Autodesk Inventor part; units mm, degrees
ref_plane "YZ Plane" through (0, 0, 0) normal (1, 0, 0) x (0, 1, 0)
ref_plane "XZ Plane" through (0, 0, 0) normal (0, 1, 0) x (-1, 0, 0)
ref_plane "XY Plane" through (0, 0, 0) normal (0, 0, 1) x (1, 0, 0)
sketch "Sketch1" plane through (0, 0, 0) normal (0, 1, 0) x (-1, 0, 0)
  line L0 (-90.805, 38.735) -> (90.805, 38.735)
  line L1 (90.805, 38.735) -> (90.805, -38.735)
  line L2 (90.805, -38.735) -> (-90.805, -38.735)
  line L3 (-90.805, -38.735) -> (-90.805, 38.735)
  line L4 (-90.805, 38.735) -> (90.805, -38.735) construction
  line L5 (90.805, 38.735) -> (-90.805, -38.735) construction
  line L6 (96.52, 43.18) -> (-96.52, 43.18)
  line L7 (-96.52, 43.18) -> (-96.52, -43.18)
  line L8 (-96.52, -43.18) -> (96.52, -43.18)
  line L9 (96.52, -43.18) -> (96.52, 43.18)
  line L10 (96.52, 43.18) -> (-96.52, -43.18) construction
  line L11 (-96.52, 43.18) -> (96.52, -43.18) construction
  point P0 (0, 0)
  dimension "d0" = 181.61
  dimension "d1" = 77.47
  dimension "d2" = 193.04
  dimension "d3" = 86.36
extrude "Extrusion1" add sketch "Sketch1" against normal blind 5.08 contours L0 L1 L2 L3 | L9 L8 L7 L6
extrude "Extrusion2" add sketch "Sketch1" along normal blind 83.566
sketch "Sketch2" plane through (-96.52, -5.08, 43.18) normal (0, 0, 1) x (1, 0, 0)
  line L0 (187.325, 88.646) -> (5.715, 88.646)
  line L1 (193.04, 88.646) -> (193.04, 0)
  line L2 (7.62, 82.423) -> (185.42, 82.423)
  line L3 (185.42, 82.423) -> (185.42, 6.223)
  line L4 (185.42, 6.223) -> (7.62, 6.223)
  line L5 (7.62, 6.223) -> (7.62, 82.423)
  line L6 (185.42, 50.673) -> (185.42, 37.973)
  line L7 (7.62, 37.973) -> (7.62, 50.673)
  line L8 (90.17, 82.423) -> (102.87, 82.423)
  line L9 (102.87, 6.223) -> (90.17, 6.223)
  line L10 (7.62, 50.673) -> (85.5215, 50.673)
  line L11 (107.5185, 50.673) -> (185.42, 50.673)
  line L12 (90.17, 6.223) -> (90.17, 33.3245)
  line L13 (90.17, 55.3215) -> (90.17, 82.423)
  line L14 (185.42, 37.973) -> (107.5185, 37.973)
  line L15 (85.5215, 37.973) -> (7.62, 37.973)
  line L16 (102.87, 82.423) -> (102.87, 55.3215)
  line L17 (102.87, 33.3245) -> (102.87, 6.223)
  arc A0 (90.17, 55.3215) -> (85.5215, 50.673) centre (96.52, 44.323) ccw
  arc A1 (107.5185, 50.673) -> (102.87, 55.3215) centre (96.52, 44.323) ccw
  arc A2 (85.5215, 37.973) -> (90.17, 33.3245) centre (96.52, 44.323) ccw
  arc A3 (102.87, 33.3245) -> (107.5185, 37.973) centre (96.52, 44.323) ccw
  line L18 (7.62, 82.423) -> (13.97, 82.423)
  line L19 (13.97, 82.423) -> (13.97, 76.073)
  line L20 (13.97, 76.073) -> (7.62, 76.073)
  line L21 (7.62, 76.073) -> (7.62, 82.423)
  line L22 (185.42, 82.423) -> (179.07, 82.423)
  line L23 (179.07, 82.423) -> (179.07, 76.073)
  line L24 (179.07, 76.073) -> (185.42, 76.073)
  line L25 (185.42, 76.073) -> (185.42, 82.423)
  line L26 (185.42, 6.223) -> (179.07, 6.223)
  line L27 (179.07, 6.223) -> (179.07, 12.573)
  line L28 (179.07, 12.573) -> (185.42, 12.573)
  line L29 (185.42, 12.573) -> (185.42, 6.223)
  line L30 (7.62, 6.223) -> (13.97, 6.223)
  line L31 (13.97, 6.223) -> (13.97, 12.573)
  line L32 (13.97, 12.573) -> (7.62, 12.573)
  line L33 (7.62, 12.573) -> (7.62, 6.223)
  line L34 (13.97, 6.223) -> (90.17, 33.3245)
  line L35 (85.5215, 37.973) -> (7.62, 12.573)
  line L36 (85.5215, 50.673) -> (7.62, 76.073)
  line L37 (13.97, 82.423) -> (90.17, 55.3215)
  line L38 (102.87, 55.3215) -> (179.07, 82.423)
  line L39 (185.42, 76.073) -> (107.5185, 50.673)
  line L40 (107.5185, 37.973) -> (185.42, 12.573)
  line L41 (179.07, 6.223) -> (102.87, 33.3245)
  point P0 (96.52, 5.08)
  point P1 (96.52, 88.646)
  point P2 (193.04, 44.323)
  point P3 (13.97, 82.423)
  point P4 (13.97, 6.223)
  dimension "d8" = 177.8
  dimension "d9" = 76.2
  dimension "d11" = 12.7
  dimension "d12" = 12.7
  dimension "d13" = 6.35
  dimension "d14" = 6.35
  dimension "d15" = 6.35
  dimension "d16" = 6.35
  dimension "d17" = 6.35
  dimension "d18" = 6.35
  dimension "d19" = 6.35
  dimension "d20" = 6.35
extrude "Extrusion3" cut sketch "Sketch2" against normal through all contours L2 L13 L37 | L36 L10 L5 | L2 L38 L16 | L15 L35 L5 | L39 L3 L11 | L12 L4 L34 | L3 L40 L14 | L17 L41 L4
sketch "Sketch3" plane through (96.52, -5.08, 43.18) normal (1, 0, 0) x (0, 0, -1)
  line L0 (81.915, 88.646) -> (4.445, 88.646)
  line L1 (86.36, 0) -> (86.36, 88.646)
  line L2 (81.915, 5.08) -> (81.915, 88.646)
  line L3 (4.445, 83.058) -> (81.915, 83.058)
  line L4 (81.915, 83.058) -> (81.915, 5.588)
  line L5 (81.915, 5.588) -> (4.445, 5.588)
  line L6 (4.445, 5.588) -> (4.445, 83.058)
  circle A0 centre (43.18, 44.323) radius 12.7
  line L7 (81.915, 50.673) -> (81.915, 37.973)
  line L8 (4.445, 37.973) -> (4.445, 50.673)
  line L9 (36.83, 83.058) -> (49.53, 83.058)
  line L10 (49.53, 5.588) -> (36.83, 5.588)
  line L11 (4.445, 50.673) -> (32.1815, 50.673)
  line L12 (54.1785, 50.673) -> (81.915, 50.673)
  line L13 (36.83, 5.588) -> (36.83, 33.3245)
  line L14 (36.83, 55.3215) -> (36.83, 83.058)
  line L15 (81.915, 37.973) -> (54.1785, 37.973)
  line L16 (32.1815, 37.973) -> (4.445, 37.973)
  line L17 (49.53, 83.058) -> (49.53, 55.3215)
  line L18 (49.53, 33.3245) -> (49.53, 5.588)
  line L19 (4.445, 83.058) -> (17.145, 83.058)
  line L20 (17.145, 83.058) -> (17.145, 70.358)
  line L21 (17.145, 70.358) -> (4.445, 70.358)
  line L22 (4.445, 70.358) -> (4.445, 83.058)
  line L23 (81.915, 83.058) -> (69.215, 83.058)
  line L24 (69.215, 83.058) -> (69.215, 70.358)
  line L25 (69.215, 70.358) -> (81.915, 70.358)
  line L26 (81.915, 70.358) -> (81.915, 83.058)
  line L27 (4.445, 5.588) -> (17.145, 5.588)
  line L28 (17.145, 5.588) -> (17.145, 18.288)
  line L29 (17.145, 18.288) -> (4.445, 18.288)
  line L30 (4.445, 18.288) -> (4.445, 5.588)
  line L31 (81.915, 5.588) -> (69.215, 5.588)
  line L32 (69.215, 5.588) -> (69.215, 18.288)
  line L33 (69.215, 18.288) -> (81.915, 18.288)
  line L34 (81.915, 18.288) -> (81.915, 5.588)
  line L35 (17.145, 5.588) -> (36.83, 33.3245)
  line L36 (32.1815, 37.973) -> (4.445, 18.288)
  line L37 (69.215, 5.588) -> (49.53, 33.3245)
  line L38 (54.1785, 37.973) -> (81.915, 18.288)
  line L39 (49.53, 55.3215) -> (69.215, 83.058)
  line L40 (54.1785, 50.673) -> (81.915, 70.358)
  line L41 (36.83, 55.3215) -> (17.145, 83.058)
  line L42 (32.1815, 50.673) -> (4.445, 70.358)
  point P0 (43.18, 5.08)
  point P1 (43.18, 88.646)
  point P2 (86.36, 44.323)
  dimension "d24" = 25.4
  dimension "d23" = 77.47
  dimension "d25" = 12.7
  dimension "d26" = 12.7
  dimension "d27" = 12.7
  dimension "d28" = 12.7
  dimension "d29" = 12.7
  dimension "d30" = 12.7
  dimension "d31" = 12.7
  dimension "d32" = 12.7
  dimension "d33" = 12.7
  dimension "d34" = 12.7
extrude "Extrusion4" cut sketch "Sketch3" against normal through all contours L38 L15 L2 | L5 L18 L37 | L12 L40 L2 | L5 L35 L13 | L36 L6 L16 | L17 L3 L39 | L11 L6 L42 | L41 L3 L14
properties part number "BatteryHolder"
Could you check a few things on this model? Use its own coordinates, in mm. A direction names the side the tool comes from. Coordinates: 2 decimals unless noted, no trailing zeros. Order: outer loops, then holes, each group sorted by start corner. A loop starts at its lowest first (then second) coordinate and runs counter-clockwise, first axis right, second up. Notation, with made-up numbers: M -33.5,18 L -23.5,18 A24 ccw -23.5,50 Z; hole C 17.5,-29.5 d3. An arc over 180 degrees is marked long. Use a Markdown table: item, result. Add a question column.
Q1. If I drill on L1, parallel to X at y = 35, z = 31 (3 decimals); L2, parallel to Z at x = -29.5, y = 25 (3 decimals); L3, parallel to Y at x = -22, z = -39, over which ranges is the centre line in solid material (lowest first)?
Q2. I want a section at A-A on y = 35. List the corners of the cut face in (x, z) for me (3 decimals).
Q3. We'd pull the mould along Z, two halves only. Please class faces 3 (the flat face through (94, 15, -6.35)), 4 (the flat face through (-45, 14.5, 41)): pulls with the +Z half, pulls with the -Z half, needs draft (parallel to the pull), parting line crosses it, or undercut.
Q4. I'm going to push flat-ended pins straight in: pin 1 (5 mm diameter, centred on x = -52.5, y = 47, fed in from -Z); pin 2 (5 mm diameter, centred on x = 67.5, z = 3.5, fed in from +Y). Where does each tip first touch, or does it pass through?
Q5. I want a section at C-C on z = -16.5. Give the number of separate pieces and of enclosed holes in the cut face, then the cut area to 3 significant figures.
Q6. I want a section at B-B on z = -3.5. List the corners of the cut face in (x, y) for me (3 decimals), then the cut area to 3 significant figures.
Q7. Which directions (+Z, -Z, +X, -X, +Y, -Y) give clear straight access to the entire face, cutting with the end or side of a thin tool? Please do faces 1 (the flat face through (-49.404, 58.115, 40.989)), 2 (the flat face through (-93.622, 55.298, -24.673)).
Checked values:
| question | item | result |
|---|---|---|
| 1 | L1 | -96.52 to -90.805, 90.805 to 96.52 |
| 1 | L2 | -43.18 to -38.735, 38.735 to 43.18 |
| 1 | L3 | -5.08 to 1.14, 22.68 to 29.31, 32.89 to 45.59, 49.18 to 55.81, 77.34 to 83.57 |
| 2 | outline | M -96.52,-43.18 L 96.52,-43.18 L 96.52,43.18 L -96.52,43.18 Z; hole M -90.805,-38.735 L 90.805,-38.735 L 90.805,38.735 L -90.805,38.735 Z |
| 3 | face 3 | undercut |
| 3 | face 4 | needs draft |
| 4 | pin 1 | z = -43.18 |
| 4 | pin 2 | y = 0 |
| 5 | separate pieces | 9 |
| 5 | enclosed holes | 0 |
| 5 | area | 1,540 mm² |
| 6 | outline | M -96.52,-5.08 L 96.52,-5.08 L 96.52,83.566 L 90.805,83.566 L 90.805,0 L -90.805,0 L -90.805,83.566 L -96.52,83.566 Z |
| 6 | area | 1,940 mm² |
| 7 | face 1 | +Z, -Z |
| 7 | face 2 | +X, -X |
